```python
from build123d import *

# Parameters (mm, degrees)
SKETCH_1_R          = 17.5
SKETCH_1_R_2        = 12.5
CUT_EXTRUDE_3_REACH = 483.521
SKETCH_3_R          = 17.5
SKETCH_3_R_2        = 12.5


with BuildPart() as part:
    # 扫描1: sweep along a path in 草图2
    with BuildLine(Plane(origin=(0, 0, 0), x_dir=(1, 0, 0), z_dir=(0, 1, 0))) as sweep_1_path:
        Line((0, 0), (-450, 0))
        ThreePointArc((-450, 0), (-485.355339059, 14.644660941), (-500, 50))
        Line((-500, 50), (-500, 400))
    # 草图1 → 扫描1 (sweep)
    with BuildSketch(Plane(origin=(0, 0, 0), x_dir=(0, 0, -1), z_dir=(1, 0, 0))):
        Circle(SKETCH_1_R)
        Circle(SKETCH_1_R_2, mode=Mode.SUBTRACT)
    sweep(path=sweep_1_path.line)

    # 草图3 → 切除-拉伸3 (cut, up to next)
    with BuildSketch(Plane(origin=(-250, 0, 0), x_dir=(0, 0, -1), z_dir=(1, 0, 0)), mode=Mode.PRIVATE) as cut_extrude_3_sk1:
        with Locations(Location((0, 0, 0), (0, 0, 180))):
            Circle(SKETCH_3_R)
        with Locations(Location((0, 0, 0), (0, 0, 180))):
            Circle(SKETCH_3_R_2, mode=Mode.SUBTRACT)
    cut_extrude_3_tool1 = extrude(cut_extrude_3_sk1.sketch, amount=CUT_EXTRUDE_3_REACH, mode=Mode.PRIVATE) & part.part
    add(cut_extrude_3_tool1.solids().sort_by_distance((-250, 0, -17.005025))[0], mode=Mode.SUBTRACT)


solid = part.part
```
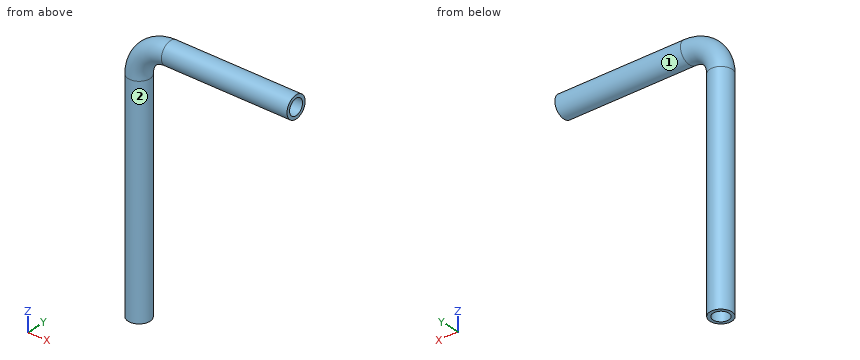
Geometry check sheet. Reference: the model listing, model coordinates, mm. Face numbers are marked on the shaded views. A direction names the side the tool comes from. Round coordinates to 2 decimals unless told otherwise and drop trailing zeros. Loops run counter-clockwise (first coordinate to the right, second up) from the corner with the lowest first, then second, coordinate; pieces in that order, holes last. Notation, with made-up numbers: (83.5, 13) -> (132.5, 13) arc R25 ccw to (132.5, 43) -> close; hole circle Ø6 at (84, 42). An arc over 180 degrees is marked (long way). Use a Markdown table: item, result.
(1) Sectioned sample at C-C (z = -364). Enter the section's corners in (x, y).
Calculated:
| item | result |
|---|---|
| outline | circle Ø35 at (-500, 0); hole circle Ø25 at (-500, 0) |
(2) Scan lines: probe 1 along X at (y, z) = (0, -289); probe 2 along Z at (x, y) = (-357, 0). Record each from-to range of solid material in increasing order.
Calculated:
| item | result |
|---|---|
| probe 1 | -517.5 to -512.5, -487.5 to -482.5 |
| probe 2 | -17.5 to -12.5, 12.5 to 17.5 |
(3) Sectioned sample at B-B (x = -279). Enter the section's corners in (y, z), then the cut area to 3 significant figures.
Calculated:
| item | result |
|---|---|
| outline | circle Ø35 at (0, 0); hole circle Ø25 at (0, 0) |
| area | 471 mm² |
(4) Sectioned sample at A-A (y = 0). Enter the section's corners in (x, z), then the cut area to 3 significant figures.
Calculated:
| item | result |
|---|---|
| outline | (-517.5, -400) -> (-512.5, -400) -> (-512.5, -50) arc R62.5 cw to (-450, 12.5) -> (-250, 12.5) -> (-250, 17.5) -> (-450, 17.5) arc R67.5 ccw to (-517.5, -50) -> close; (-487.5, -400) -> (-482.5, -400) -> (-482.5, -50) arc R32.5 cw to (-450, -17.5) -> (-250, -17.5) -> (-250, -12.5) -> (-450, -12.5) arc R37.5 ccw to (-487.5, -50) -> close |
| area | 6,290 mm² |
(5) Set-up check for the marked faces 1 and 2: record each of +Z, -Z, +X, -X, +Y, -Y from which the full face is reachable in a straight line by a thin tool's end or side.
Calculated:
| item | result |
|---|---|
| face 1 | +X |
| face 2 | -Z |
(6) Go/stop test with flat-tipped pins: P1, Ø5, axis at x = -403.5, y = -13.5, coming from the +Z side; P2, Ø2, axis at y = -12, z = -192.5, coming from the -X side; P3, Ø12, axis at y = 0.5, z = -351, coming from the +X side. Record where each tip stops, or that it passes through.
Calculated:
| item | result |
|---|---|
| P1 | z = 13.61 |
| P2 | x = -513.61 |
| P3 | x = -482.5 |
